Verification items for the finished model (mm, model axes). A direction names the side the tool comes from. Coordinates: 2 decimals unless noted, no trailing zeros. Write each loop counter-clockwise with the first axis right and the second up, starting at its lowest first coordinate (ties: lowest second). Pieces come first, ordered by that corner, then holes. Notation, with made-up numbers: M 26,79.25 L 74,79.25 A37 cw 74,115.25 Z; hole C 88,22 d6. An arc over 180 degrees is marked long. Answer in a Markdown table with one row per item.
from build123d import *

# Parameters (mm, degrees)
SKETCH4_W           = 20
SKETCH4_H           = 120
BOSS_EXTRUDE4_DEPTH = 10
SKETCH5_R           = 2.1
CUT_EXTRUDE1_DEPTH  = 10
SKETCH6_W           = 20
SKETCH6_H           = 50
BOSS_EXTRUDE5_DEPTH = 50
SKETCH7_W           = 40.5
SKETCH7_H           = 20.5
CUT_EXTRUDE2_DEPTH  = 20
SKETCH8_R           = 2.6
CUT_EXTRUDE3_DEPTH  = 50
SKETCH9_W           = 4.75
SKETCH9_H           = 30
SKETCH9_W_2         = 5
BOSS_EXTRUDE6_DEPTH = 40
CUT_EXTRUDE4_DEPTH  = 40
BOSS_EXTRUDE7_START = -29.75
SKETCH11_W          = 5
SKETCH11_H          = 30
BOSS_EXTRUDE7_DEPTH = 29.75
SKETCH12_R          = 2.1
CUT_EXTRUDE5_DEPTH  = 5
CHAMFER1_SIZE       = 20
CHAMFER2_SIZE       = 10


with BuildPart() as part:
    # Sketch4 → Boss-Extrude4 (new body)
    with BuildSketch(Plane(origin=(0, 0, 0), x_dir=(1, 0, 0), z_dir=(0, 1, 0))):
        with Locations((10, 60)):
            Rectangle(SKETCH4_W, SKETCH4_H)
    extrude(amount=BOSS_EXTRUDE4_DEPTH)

    # Sketch5 → Cut-Extrude1 (cut)
    with BuildSketch(Plane(origin=(0, 10, 0), x_dir=(1, 0, 0), z_dir=(0, 1, 0))):
        with Locations(Location((10, 105, 0), (0, 0, 270))):
            Circle(SKETCH5_R)
        with Locations(Location((10, 15, 0), (0, 0, 270))):
            Circle(SKETCH5_R)
    extrude(amount=-CUT_EXTRUDE1_DEPTH, mode=Mode.SUBTRACT)

    # Sketch6 → Boss-Extrude5 (add)
    with BuildSketch(Plane(origin=(0, 10, 0), x_dir=(1, 0, 0), z_dir=(0, 1, 0))):
        with Locations((10, 70)):
            Rectangle(SKETCH6_W, SKETCH6_H)
    extrude(amount=BOSS_EXTRUDE5_DEPTH)

    # Sketch7 → Cut-Extrude2 (cut)
    with BuildSketch(Plane.ZY):
        with Locations((-70, 44.85)):
            Rectangle(SKETCH7_W, SKETCH7_H)
    extrude(amount=-CUT_EXTRUDE2_DEPTH, mode=Mode.SUBTRACT)

    # Sketch8 → Cut-Extrude3 (cut, symmetric)
    with BuildSketch(Plane.XY.offset(-90.25)):
        with Locations((10, 44.85)):
            Circle(SKETCH8_R)
    extrude(amount=CUT_EXTRUDE3_DEPTH, both=True, mode=Mode.SUBTRACT)

    # Sketch9 → Boss-Extrude6 (add)
    with BuildSketch(Plane.ZY):
        with Locations((-47.375, 45)):
            Rectangle(SKETCH9_W, SKETCH9_H)
        with Locations((-72.25, 45)):
            Rectangle(SKETCH9_W_2, SKETCH9_H)
    extrude(amount=BOSS_EXTRUDE6_DEPTH)

    # Sketch10 → Cut-Extrude4 (cut)
    with BuildSketch(Plane(origin=(0, 0, -74.75), x_dir=(-1, 0, 0), z_dir=(0, 0, -1))):
        with BuildLine():
            Line((33.5, 42.3), (9.5, 42.3))
            ThreePointArc((9.5, 42.3), (6.9, 44.9), (9.5, 47.5))
            Line((9.5, 47.5), (33.5, 47.5))
            ThreePointArc((33.5, 47.5), (36.1, 44.9), (33.5, 42.3))
        make_face()
    extrude(amount=-CUT_EXTRUDE4_DEPTH, mode=Mode.SUBTRACT)

    # Sketch11 → Boss-Extrude7 (add)
    with BuildSketch(Plane(origin=(0, 0, -74.75), x_dir=(-1, 0, 0), z_dir=(0, 0, -1)).offset(BOSS_EXTRUDE7_START)):
        with Locations((40.5, 45)):
            Rectangle(SKETCH11_W, SKETCH11_H)
    extrude(amount=BOSS_EXTRUDE7_DEPTH)

    # Sketch12 → Cut-Extrude5 (cut)
    with BuildSketch(Plane.ZY.offset(43)):
        with Locations((-59.875, 45)):
            Circle(SKETCH12_R)
    extrude(amount=-CUT_EXTRUDE5_DEPTH, mode=Mode.SUBTRACT)

    # Chamfer1
    chamfer1_edges = [part.edges().sort_by_distance(p)[0] for p in [
        (0, 30, -47.375),
        (0, 30, -72.25),
    ]]
    chamfer(chamfer1_edges, length=CHAMFER1_SIZE)

    # Chamfer2
    chamfer2_edges = [part.edges().sort_by_distance(p)[0] for p in [
        (0, 57.55, -74.75),
        (0, 22.3, -74.75),
    ]]
    chamfer(chamfer2_edges, length=CHAMFER2_SIZE)


solid = part.part
1) Sectioned sample at B-B (x = -25). Record the cut outline in (y, z).
Response values:
| item | result |
|---|---|
| outline | M 30,-74.75 L 42.3,-74.75 L 42.3,-69.75 L 30,-69.75 Z; M 30,-49.75 L 42.3,-49.75 L 42.3,-45 L 30,-45 Z; M 47.5,-74.75 L 60,-74.75 L 60,-69.75 L 47.5,-69.75 Z; M 47.5,-49.75 L 60,-49.75 L 60,-45 L 47.5,-45 Z |
2) Tool access check on faces 1 (the face through (-39, 30, -63)), 2 (the face through (0, 45, -72)), 3 (the face through (-6.9, 44.8, -72.3)), 4 (the face through (10, 10, -23)). Record the directions out of +Z, -Z, +X, -X, +Y, -Y that give a thin tool (end or side, any length) a straight path to the whole face; none if there is none.
Response values:
| item | result |
|---|---|
| face 1 | +Z, -Z, -X, -Y |
| face 2 | +X |
| face 3 | +Z, -Z |
| face 4 | +Z, +X, -X, +Y |
3) Thickness scan on L1, parallel to Z at x = -6, y = 50; L2, parallel to Z at x = 6, y = 51; L3, parallel to Y at x = 10, z = -93.75. Record the ranges inside material, lowest first. Write a range as [from, to].
Response values:
| item | result |
|---|---|
| L1 | z = [-74.75, -69.75], [-49.75, -45] |
| L2 | z = [-95, -90.25], [-49.75, -45] |
| L3 | y = [0, 42.25], [47.45, 60] |
4) Depth check by flat-ended pin: pin 1 (1.5 mm diameter, centred on x = 5, y = 16, fed in from -Z); pin 2 (2.5 mm diameter, centred on x = -21, z = -48, fed in from -Y); pin 3 (11.5 mm diameter, centred on x = -34.5, z = -53.5, fed in from -Y). Enter the tip coordinate at first touch or a pass-through.
Response values:
| item | result |
|---|---|
| pin 1 | stops at z = -95 |
| pin 2 | stops at y = 29.75 |
| pin 3 | stops at y = 30 |
5) Sectioned sample at A-A (z = -82). Record the cut outline in (x, y).
Response values:
| item | result |
|---|---|
| outline | M -2.75,12.75 L 0,10 L 0,0 L 20,0 L 20,34.6 L -2.75,34.6 Z; M -2.75,55.1 L 20,55.1 L 20,60 L -2.75,60 Z |
6) Release check for a two-part mould opening along X. For faces 5 (the face through (0, 58, -60)), 6 (the face through (-10, 20, -47)), 7 (the face through (10, 35, -95)) record: +X half, -X half, draft (parallel to the pull), parting line (faces both ways), or undercut.
Response values:
| item | result |
|---|---|
| face 5 | undercut |
| face 6 | -X half |
| face 7 | draft |
7) Sectioned sample at C-C (y = 12). Record the cut outline in (x, z).
Response values:
| item | result |
|---|---|
| outline | M -2,-82.75 L 0,-84.75 L 0,-95 L 20,-95 L 20,-45 L -2,-45 L -2,-49.75 L 0,-49.75 L 0,-69.75 L -2,-69.75 Z |
8) Sectioned sample at D-D (z = -65). Record the cut outline in (x, y), then the cut area to 3 significant figures.
Response values:
| item | result |
|---|---|
| outline | M -43,30 L -38,30 L -38,60 L -43,60 Z; M 0,0 L 20,0 L 20,34.6 L 0,34.6 Z; M 0,55.1 L 20,55.1 L 20,60 L 0,60 Z |
| area | 940 mm² |
